Verification items for the finished model (mm, model axes). A direction names the side the tool comes from. Coordinates: 2 decimals unless noted, no trailing zeros. Order: outer loops, then holes, each group sorted by start corner. A loop starts at its lowest first (then second) coordinate and runs counter-clockwise, first axis right, second up. Notation, with made-up numbers: M 66.25,51 L 75.25,51 A29 ccw 75.25,85 Z; hole C 36.25,45.25 d5. An arc over 180 degrees is marked long. Answer as a JSON object with one key per item and string values. Group by question number.
(1) Access from +Z, -Z, +X, -X, +Y, -Y to the whole of each face (thin tool, end or side, straight path). Record for faces 1 (the face through (60, -9, 0)), 2 (the face through (1, -16, -112.5)), 3 (the face through (-47, -31, -98)), 4 (the face through (23, -1, -29)), 5 (the face through (-1, -16, -111)).
(2) Cross-section at C-C (z = -49). Enter the section's corners in (x, y), plus the area to 4 significant figures.
(3) Gauge pin test, flat ends, axial feed: pin 1 Ø10 at (x, y) = (3.5, -12) entering from +Z; pin 2 Ø3 at (y, z) = (-25, -11.5) entering from -X; pin 3 Ø6.5 at (x, z) = (-63, -78) entering from -Y. Record the tip position at first contact, or that the pin passes through.
(4) Cross-section at A-A (z = -12.5). Enter the section's corners in (x, y), plus the area to 3 significant figures.
(5) Cross-section at B-B (y = -22). Enter the section's corners in (x, z).
(6) Cross-section at D-D (x = -4.5). Enter the section's corners in (y, z), plus the area to 4 significant figures.
(7) Mould release check, pull along Y, two halves, no side actions. Record for faces 6 (the face through (-27, -1, -1)), 7 (the face through (59, -16, -55)), 8 (the face through (-64, -1.5, -55)), 9 (the face through (0, -30, -102)): released by +Y, released by -Y, zero draft, split by the parting line, or undercut.
(8) Material ranges on line 1 (X direction, y = -19.5, z = -99); line 2 (Y direction, x = -56, z = -79); line 3 (Y direction, x = -23.5, z = -58.5), recorded low to high.
from build123d import *

# Parameters (mm, degrees)
PAD_DEPTH        = 112.5
SKETCH002_W      = 118
SKETCH002_H      = 28.5
POCKET_DEPTH     = 111
SKETCH003_W      = 96
SKETCH003_H      = 30
POCKET001_DEPTH  = 100
SKETCH004_R      = 1.9
PAD001_DEPTH     = 20
SKETCH005_W      = 50
SKETCH005_H      = 50
POCKET002_DEPTH  = 30
FILLET_R         = 5
FILLET001_R      = 1
CHAMFER_SIZE2    = 50
CHAMFER_SIZE     = 1
CHAMFER001_SIZE  = 1.5
CHAMFER002_SIZE  = 1.35
CHAMFER003_SIZE2 = 15
CHAMFER003_SIZE  = 0.5
SKETCH006_W      = 6
SKETCH006_H      = 28.5
POCKET003_DEPTH  = 5


with BuildPart() as part:
    # Sketch → Pad (new body)
    with BuildSketch(Plane.XY):
        Polygon((-67.5, 0), (67.5, 0), (67.5, -1.5), (60.5, -1.5), (60.5, -31.5), (-60.5, -31.5), (-60.5, -1.5), (-67.5, -1.5), align=None)
    extrude(amount=-PAD_DEPTH)

    # Sketch002 → Pocket (cut)
    with BuildSketch(Plane.XY):
        with Locations((0, -15.75)):
            Rectangle(SKETCH002_W, SKETCH002_H)
    extrude(amount=-POCKET_DEPTH, mode=Mode.SUBTRACT)

    # Sketch003 → Pocket001 (cut)
    with BuildSketch(Plane.XY):
        with Locations((0, -25)):
            Rectangle(SKETCH003_W, SKETCH003_H)
    extrude(amount=-POCKET001_DEPTH, mode=Mode.SUBTRACT)

    # Sketch004 → Pad001 (join)
    with BuildSketch(Plane.XY):
        with Locations((-67, -0.75)):
            Circle(SKETCH004_R)
        with Locations((67, -0.75)):
            Circle(SKETCH004_R)
    extrude(amount=-PAD001_DEPTH)

    # Sketch005 → Pocket002 (cut)
    with BuildSketch(Plane.XY):
        Rectangle(SKETCH005_W, SKETCH005_H)
    extrude(amount=-POCKET002_DEPTH, mode=Mode.SUBTRACT)

    # Fillet
    fillet_edges = [part.edges().sort_by_distance(p)[0] for p in [
        (-25, -0.75, 0),
        (25, -0.75, 0),
        (25, -0.75, -30),
        (-25, -0.75, -30),
        (-48, -30.75, 0),
        (48, -30.75, 0),
        (48, -30.75, -100),
        (-48, -30.75, -100),
    ]]
    fillet(fillet_edges, radius=FILLET_R)

    # Fillet001
    fillet001_edges = [part.edges().sort_by_distance(p)[0] for p in [
        (-60.5, -1.5, -56.25),
        (-60.5, -31.5, -56.25),
        (60.5, -31.5, -56.25),
        (60.5, -1.5, -56.25),
    ]]
    fillet(fillet001_edges, radius=FILLET001_R)

    # Chamfer
    chamfer_edges = [part.edges().sort_by_distance(p)[0] for p in [
        (67.5, -0.75, -112.5),
        (-67.5, -0.75, -112.5),
    ]]
    chamfer_side = part.faces().sort_by_distance((0, -15.664499, -112.5))[0]
    chamfer(chamfer_edges, length=CHAMFER_SIZE, length2=CHAMFER_SIZE2, reference=chamfer_side)

    # Chamfer001
    chamfer001_edges = [part.edges().sort_by_distance(p)[0] for p in [
        (-66.5, -0.75, -112.5),
        (66.5, -0.75, -112.5),
    ]]
    chamfer(chamfer001_edges, length=CHAMFER001_SIZE)

    # Chamfer002
    chamfer002_edges = [part.edges().sort_by_distance(p)[0] for p in [
        (-68.9, -0.75, -20),
        (67.382853, 1.111028, -20),
    ]]
    chamfer(chamfer002_edges, length=CHAMFER002_SIZE)

    # Chamfer003
    chamfer003_edges = [part.edges().sort_by_distance(p)[0] for p in [
        (0, 0, -112.5),
    ]]
    chamfer003_side = part.faces().sort_by_distance((0, -15.693743, -112.5))[0]
    chamfer(chamfer003_edges, length=CHAMFER003_SIZE, length2=CHAMFER003_SIZE2, reference=chamfer003_side)

    # Sketch006 (on Face46 of Chamfer003) → Pocket003 (cut)
    with BuildSketch(Plane.XY.offset(-111)):
        with Locations((56, -15.75)):
            Rectangle(SKETCH006_W, SKETCH006_H)
        with Locations((-56, -15.75)):
            Rectangle(SKETCH006_W, SKETCH006_H)
    extrude(amount=-POCKET003_DEPTH, mode=Mode.SUBTRACT)


solid = part.part
Taken from the geometry:
{
 "1": {"face 1": "+Z, +X, -X, +Y, -Y", "face 2": "-Z, +X, -X, +Y, -Y", "face 3": "+Z, -Y", "face 4": "+Z, +Y, -Y", "face 5": "+Z"},
 "2": {"outline": "M -67.5,-1.5 L -61.5,-1.5 A1 cw -60.5,-2.5 L -60.5,-30.5 A1 ccw -59.5,-31.5 L -48,-31.5 L -48,-30 L -59,-30 L -59,-1.5 L 59,-1.5 L 59,-30 L 48,-30 L 48,-31.5 L 59.5,-31.5 A1 ccw 60.5,-30.5 L 60.5,-2.5 A1 cw 61.5,-1.5 L 67.5,-1.5 L 67.5,0 L -67.5,0 Z", "area": "325.5 mm²"},
 "3": {"pin 1": "stops at z = -111", "pin 2": "stops at x = -60.5", "pin 3": "stops at y = -31.47"},
 "4": {"outline": "M -65.25,-1.5 L -61.5,-1.5 A1 cw -60.5,-2.5 L -60.5,-30.5 A1 ccw -59.5,-31.5 L -48,-31.5 L -48,-30 L -59,-30 L -59,-1.5 L -25,-1.5 L -25,0 L -65.25,0 A1.9 ccw long Z; M 25,-1.5 L 59,-1.5 L 59,-30 L 48,-30 L 48,-31.5 L 59.5,-31.5 A1 ccw 60.5,-30.5 L 60.5,-2.5 A1 cw 61.5,-1.5 L 65.25,-1.5 A1.9 ccw long 65.25,0 L 25,0 Z", "area": "266 mm²"},
 "5": {"outline": "M -60.5,-112.5 L -59,-112.5 L -59,0 L -60.5,0 Z; M -53,-112.5 L 53,-112.5 L 53,-111 L -53,-111 Z; M 59,-112.5 L 60.5,-112.5 L 60.5,0 L 59,0 Z"},
 "6": {"outline": "M -31.5,-112.5 L -0.5,-112.5 L 0,-97.5 L 0,-30 L -1.5,-30 L -1.5,-111 L -30,-111 L -30,-100 L -31.5,-100 Z", "area": "181.5 mm²"},
 "7": {"face 6": "zero draft", "face 7": "undercut", "face 8": "released by -Y", "face 9": "undercut"},
 "8": {"line 1": "x = -60.5 to -59, 59 to 60.5", "line 2": "y = -31.5 to -30, -1.5 to 0", "line 3": "y = -1.5 to 0"}
}
